Can you work these out from the model? Positions are in its coordinate system, mm. Face numbers are marked on the shaded views. A direction names the side the tool comes from. Round coordinates to 2 decimals unless told otherwise and drop trailing zeros. Loops run counter-clockwise (first coordinate to the right, second up) from the corner with the lowest first, then second, coordinate; pieces in that order, holes last. Notation, with made-up numbers: (58, -3.5) -> (114, -3.5) arc R17 cw to (114, 14.5) -> close; hole circle Ø10 at (-21.5, 16). An arc over 180 degrees is marked (long way). Use a Markdown table: item, result.
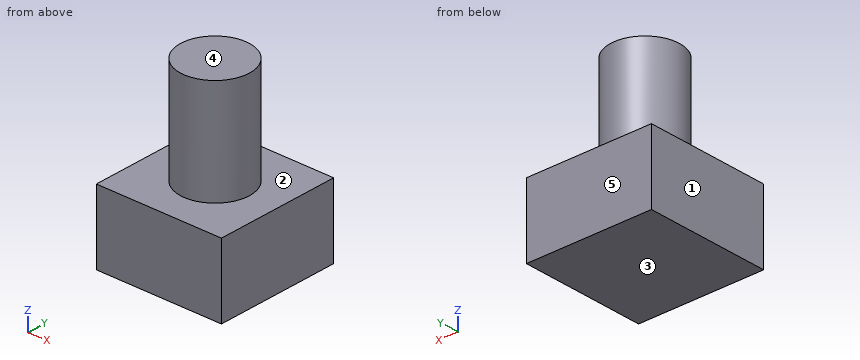
Autodesk Inventor part; units mm, degrees
ref_plane "YZ Plane" through (0, 0, 0) normal (1, 0, 0) x (0, 1, 0)
ref_plane "XZ Plane" through (0, 0, 0) normal (0, 1, 0) x (-1, 0, 0)
ref_plane "XY Plane" through (0, 0, 0) normal (0, 0, 1) x (1, 0, 0)
sketch "Sketch1" plane through (0, 0, 0) normal (0, 0, 1) x (1, 0, 0)
  circle A0 centre (0, 0) radius 1.65
  dimension "d0" = 3.3
extrude "Extrusion1" add sketch "Sketch1" along normal blind 5
sketch "Sketch2" plane through (0, 0, 0) normal (0, 0, 1) x (1, 0, 0)
  line L0 (3, -3) -> (-3, -3)
  line L1 (-3, -3) -> (-3, 3)
  line L2 (-3, 3) -> (3, 3)
  line L3 (3, 3) -> (3, -3)
  line L4 (-4.2165, 0) -> (4.1835, 0)
  line L5 (0, -4.2) -> (0, 4.2)
  point P0 (0, 0)
  point P1 (3, 0)
  point P2 (0, 3)
  dimension "d3" = 6
extrude "Extrusion2" add sketch "Sketch2" against normal blind 3.5
properties part number "Button"
1. I need wall thicknesses on line 1 (Z direction, x = 0.6, y = -2.45); line 2 (Y direction, x = -0.35, z = 4.5); line 3 (X direction, y = 0.3, z = 3.5). Which ranges of each line are inside material? Lowest first, please.
Answer sheet:
| item | result |
|---|---|
| line 1 | z = -3.5 to 0 |
| line 2 | y = -1.61 to 1.61 |
| line 3 | x = -1.62 to 1.62 |
2. I want a section at A-A (y = 0). Please give me the cut outline in (x, z).
Answer sheet:
| item | result |
|---|---|
| outline | (-3, -3.5) -> (3, -3.5) -> (3, 0) -> (1.65, 0) -> (1.65, 5) -> (-1.65, 5) -> (-1.65, 0) -> (-3, 0) -> close |
3. I want a section at C-C (z = 2). Please give me the cut outline in (x, y), plus the area to 3 significant figures.
Answer sheet:
| item | result |
|---|---|
| outline | circle Ø3.3 at (0, 0) |
| area | 8.55 mm² |
4. I want a section at D-D (x = -2.35). Please give me the cut outline in (y, z).
Answer sheet:
| item | result |
|---|---|
| outline | (-3, -3.5) -> (3, -3.5) -> (3, 0) -> (-3, 0) -> close |
5. Which directions (+Z, -Z, +X, -X, +Y, -Y) give clear straight access to the entire face, cutting with the end or side of a thin tool? Please do the marked faces 1 and 2.
Answer sheet:
| item | result |
|---|---|
| face 1 | +Z, -Z, -X, +Y, -Y |
| face 2 | +Z |
6. If we mould it in two halves opening along Z, with no side actions, what happens to the marked faces 3, 4 and 5? For each: +Z half, -Z half, draft (parallel to the pull), parting line (faces both ways), or undercut.
Answer sheet:
| item | result |
|---|---|
| face 3 | -Z half |
| face 4 | +Z half |
| face 5 | draft |
7. Will this pin go through, and if not, where does the flat tip stop? pin 1 Ø2 at (y, z) = (0, 2.5) entering from +X.
Answer sheet:
| item | result |
|---|---|
| pin 1 | stops at x = 1.65 |
